Check sheet for the drawn part. Datum: minimum x, y, z corner. Units: mm. A direction names the side the tool comes from. Round coordinates to 2 decimals unless told otherwise and drop trailing zeros. Write each loop counter-clockwise with the first axis right and the second up, starting at its lowest first coordinate (ties: lowest second). Pieces come first, ordered by that corner, then holes. Notation, with made-up numbers: (3.25, -0.75) - (34.25, -0.75) arc R18 cw to (34.25, 5.25) - close; hole circle Ø10 at (10, -20). An arc over 180 degrees is marked (long way). Answer as a JSON object with one key per item and string values. Group by question number.
1) Thickness scan on line 1 (X direction, y = 2.58, z = 1.75); line 2 (X direction, y = 1.35, z = 0.6); line 3 (Y direction, x = 2.5, z = 2.4) (1 decimal). Record the ranges inside material, lowest first.
2) Go/stop test with flat-tipped pins: pin 1 Ø1 at (y, z) = (1, 1.5) entering from -X; pin 2 Ø0.8 at (y, z) = (0.5, 2) entering from -X. Record where each tip stops, or that it passes through.
3) Section check B-B (x = 5.75). Enter the section's corners in (y, z) (3 decimals), then the cut area to 3 significant figures.
4) Section check A-A (y = 1.6). Enter the section's corners in (x, z), then the cut area to 3 significant figures.
5) Mould release check, pull along X, two halves, no side actions. Record for the marked faces 1, 2, 3 and 4: +X half, -X half, draft (parallel to the pull), parting line (faces both ways), or undercut.
6) Section check D-D (x = 1.5). Enter the section's corners in (y, z).
7) Set-up check for the marked faces 5 and 6: record each of +Z, -Z, +X, -X, +Y, -Y from which the full face is reachable in a straight line by a thin tool's end or side.
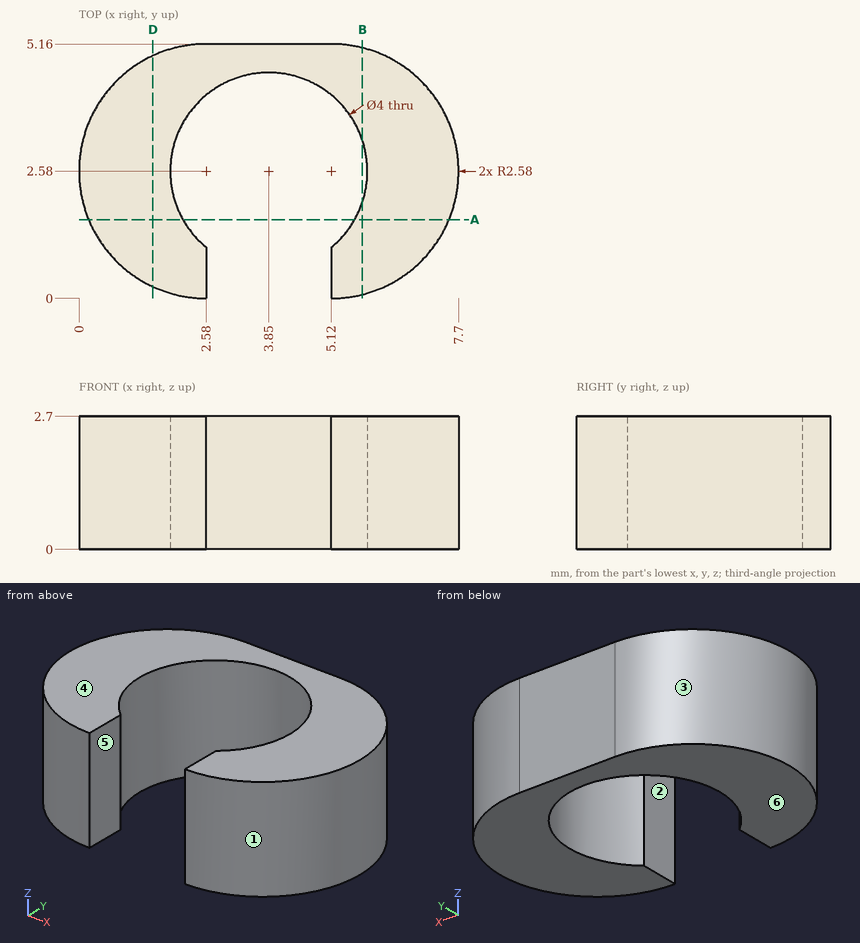
Returned:
{
 "1": {"line 1": "0 to 1.85, 5.85 to 7.7", "line 2": "0.31 to 2.27, 5.43 to 7.39", "line 3": "0 to 1.1, 4.1 to 5.2"},
 "2": {"pin 1": "x = 0.24", "pin 2": "x = 0.62"},
 "3": {"outline": "(0.078, 0) - (1.955, 0) - (1.955, 2.7) - (0.078, 2.7) - close; (3.205, 0) - (5.082, 0) - (5.082, 2.7) - (3.205, 2.7) - close", "area": "10.1 mm2"},
 "4": {"outline": "(0.19, 0) - (2.11, 0) - (2.11, 2.7) - (0.19, 2.7) - close; (5.59, 0) - (7.51, 0) - (7.51, 2.7) - (5.59, 2.7) - close", "area": "10.3 mm2"},
 "5": {"face 1": "+X half", "face 2": "undercut", "face 3": "-X half", "face 4": "draft"},
 "6": {"outline": "(0.24, 0) - (4.92, 0) - (4.92, 2.7) - (0.24, 2.7) - close"},
 "7": {"face 5": "+Z, -Z, -Y", "face 6": "-Z, +X, -X, +Y, -Y"}
}
